```python
from build123d import *

# Parameters (mm, degrees)
SKETCH2_R           = 2.246119438
BOSS_EXTRUDE1_DEPTH = 5
SKETCH1_W           = 67
SKETCH1_H           = 30
SKETCH1_R           = 6.25
SKETCH1_R_2         = 1
BOSS_EXTRUDE3_DEPTH = 5
SKETCH8_W           = 30
SKETCH8_H           = 40
BOSS_EXTRUDE4_DEPTH = 5
SKETCH9_W           = 30
SKETCH9_H           = 40
BOSS_EXTRUDE5_DEPTH = 5
SKETCH11_W          = 30
SKETCH11_H          = 5
BOSS_EXTRUDE6_DEPTH = 40
SKETCH12_W          = 30
SKETCH12_H          = 5
BOSS_EXTRUDE7_DEPTH = 40
SKETCH13_R          = 2.195864451
CUT_EXTRUDE1_DEPTH  = 5
SKETCH14_R          = 1
CUT_EXTRUDE2_DEPTH  = 5
SKETCH15_R          = 2.070506859
CUT_EXTRUDE3_DEPTH  = 5
SKETCH16_R          = 1.962714384
CUT_EXTRUDE4_DEPTH  = 5


with BuildPart() as part:
    # Sketch2 → Boss-Extrude1 (new body)
    with BuildSketch(Plane(origin=(0, 0, 0), x_dir=(0, 0, -1), z_dir=(1, 0, 0))):
        with BuildLine():
            Line((30, 0), (0, 0))
            Line((0, 0), (0, 40))
            Line((0, 40), (7.960594487, 40))
            ThreePointArc((7.960594487, 40), (14.468438583, 30), (20.976282678, 40))
            Line((20.976282678, 40), (30, 40))
            Line((30, 40), (30, 0))
        make_face()
        with Locations((14.468438583, 24.238644745)):
            Circle(SKETCH2_R, mode=Mode.SUBTRACT)
        with Locations((6.578911504, 27.652835849)):
            Circle(SKETCH2_R, mode=Mode.SUBTRACT)
        with Locations((3.414371088, 35.645771628)):
            Circle(SKETCH2_R, mode=Mode.SUBTRACT)
        with Locations((25.875565465, 35.29271224)):
            Circle(SKETCH2_R, mode=Mode.SUBTRACT)
        with Locations((22.461374361, 27.403185161)):
            Circle(SKETCH2_R, mode=Mode.SUBTRACT)
    boss_extrude1 = extrude(amount=-BOSS_EXTRUDE1_DEPTH)

    # Sketch1 → Boss-Extrude3 (add)
    with BuildSketch(Plane(origin=(0, 0, 0), x_dir=(1, 0, 0), z_dir=(0, 1, 0))):
        with Locations((33.5, 15)):
            Rectangle(SKETCH1_W, SKETCH1_H)
        with Locations(Location((33.5, 15, 0), (0, 0, 270))):
            Circle(SKETCH1_R, mode=Mode.SUBTRACT)
        with Locations(Location((42, 23.5, 0), (0, 0, 270))):
            Circle(SKETCH1_R_2, mode=Mode.SUBTRACT)
        with Locations(Location((42, 6.5, 0), (0, 0, 270))):
            Circle(SKETCH1_R_2, mode=Mode.SUBTRACT)
        with Locations(Location((25, 6.5, 0), (0, 0, 270))):
            Circle(SKETCH1_R_2, mode=Mode.SUBTRACT)
        with Locations(Location((25, 23.5, 0), (0, 0, 270))):
            Circle(SKETCH1_R_2, mode=Mode.SUBTRACT)
        with Locations(Location((53.5, 5, 0), (0, 0, 270))):
            Circle(SKETCH1_R_2, mode=Mode.SUBTRACT)
        with Locations(Location((53.5, 25, 0), (0, 0, 270))):
            Circle(SKETCH1_R_2, mode=Mode.SUBTRACT)
        with Locations(Location((13.5, 25, 0), (0, 0, 270))):
            Circle(SKETCH1_R_2, mode=Mode.SUBTRACT)
        with Locations(Location((13.5, 5, 0), (0, 0, 270))):
            Circle(SKETCH1_R_2, mode=Mode.SUBTRACT)
    extrude(amount=BOSS_EXTRUDE3_DEPTH)

    # Mirror1: Boss-Extrude1 across plane
    add(boss_extrude1.mirror(Plane(origin=(33.5, 0, 0), x_dir=(0, 0, 1), z_dir=(1, 0, 0))))

    # Sketch8 → Boss-Extrude4 (add)
    with BuildSketch(Plane.ZY.offset(5)):
        with Locations((-15, 20)):
            Rectangle(SKETCH8_W, SKETCH8_H)
    extrude(amount=-BOSS_EXTRUDE4_DEPTH)

    # Sketch9 → Boss-Extrude5 (add)
    with BuildSketch(Plane(origin=(72, 0, 0), x_dir=(0, 0, -1), z_dir=(1, 0, 0))):
        with Locations((15, 20)):
            Rectangle(SKETCH9_W, SKETCH9_H)
    extrude(amount=-BOSS_EXTRUDE5_DEPTH)

    # Sketch11 → Boss-Extrude6 (add)
    with BuildSketch(Plane(origin=(72, 0, 0), x_dir=(0, 0, -1), z_dir=(1, 0, 0))):
        with Locations((15, 37.5)):
            Rectangle(SKETCH11_W, SKETCH11_H)
    extrude(amount=BOSS_EXTRUDE6_DEPTH)

    # Sketch12 → Boss-Extrude7 (add)
    with BuildSketch(Plane.ZY.offset(5)):
        with Locations((-15, 37.5)):
            Rectangle(SKETCH12_W, SKETCH12_H)
    extrude(amount=BOSS_EXTRUDE7_DEPTH)

    # Sketch13 → Cut-Extrude1 (cut)
    with BuildSketch(Plane(origin=(72, 0, 0), x_dir=(0, 0, -1), z_dir=(1, 0, 0))):
        with Locations((4.552108339, 18.246803651)):
            Circle(SKETCH13_R)
        with Locations((7.738751357, 11.072716755)):
            Circle(SKETCH13_R)
        with Locations((15.064893737, 8.253168149)):
            Circle(SKETCH13_R)
        with Locations((22.238980633, 11.439811167)):
            Circle(SKETCH13_R)
        with Locations((25.058529239, 18.765953547)):
            Circle(SKETCH13_R)
        with Locations((21.871886221, 25.940040443)):
            Circle(SKETCH13_R)
        with Locations((14.545743841, 28.759589048)):
            Circle(SKETCH13_R)
        with Locations((7.371656945, 25.572946031)):
            Circle(SKETCH13_R)
    extrude(amount=-CUT_EXTRUDE1_DEPTH, mode=Mode.SUBTRACT)

    # Sketch14 → Cut-Extrude2 (cut)
    with BuildSketch(Plane.XZ.offset(-35)):
        with Locations(Location((82.265636432, -14.777839144, 0), (0, 0, 270))):
            Circle(SKETCH14_R)
        with Locations(Location((85.666207992, -23.170222577, 0), (0, 0, 270))):
            Circle(SKETCH14_R)
        with Locations(Location((94.347859261, -25.744114158, 0), (0, 0, 270))):
            Circle(SKETCH14_R)
        with Locations(Location((101.77312976, -20.561321027, 0), (0, 0, 270))):
            Circle(SKETCH14_R)
        with Locations(Location((102.350639356, -11.524592123, 0), (0, 0, 270))):
            Circle(SKETCH14_R)
        with Locations(Location((95.645511544, -5.438768625, 0), (0, 0, 270))):
            Circle(SKETCH14_R)
        with Locations(Location((86.706844325, -6.886599756, 0), (0, 0, 270))):
            Circle(SKETCH14_R)
    extrude(amount=-CUT_EXTRUDE2_DEPTH, mode=Mode.SUBTRACT)

    # Sketch15 → Cut-Extrude3 (cut)
    with BuildSketch(Plane.ZY.offset(5)):
        with Locations((-15.389362422, 28.629801574)):
            Circle(SKETCH15_R)
        with Locations((-23.658210405, 24.452096347)):
            Circle(SKETCH15_R)
        with Locations((-26.55108519, 15.65105417)):
            Circle(SKETCH15_R)
        with Locations((-22.373379963, 7.382206187)):
            Circle(SKETCH15_R)
        with Locations((-13.572337785, 4.489331401)):
            Circle(SKETCH15_R)
        with Locations((-5.303489803, 8.667036629)):
            Circle(SKETCH15_R)
        with Locations((-2.410615017, 17.468078806)):
            Circle(SKETCH15_R)
        with Locations((-6.588320245, 25.736926789)):
            Circle(SKETCH15_R)
    extrude(amount=-CUT_EXTRUDE3_DEPTH, mode=Mode.SUBTRACT)

    # Sketch16 → Cut-Extrude4 (cut)
    with BuildSketch(Plane.XZ.offset(-35)):
        with Locations(Location((-39.786222938, -13.841664359, 0), (0, 0, 270))):
            Circle(SKETCH16_R)
        with Locations(Location((-36.298214509, -6.315787831, 0), (0, 0, 270))):
            Circle(SKETCH16_R)
        with Locations(Location((-28.510221767, -3.460583916, 0), (0, 0, 270))):
            Circle(SKETCH16_R)
        with Locations(Location((-20.984345239, -6.948592346, 0), (0, 0, 270))):
            Circle(SKETCH16_R)
        with Locations(Location((-18.129141325, -14.736585087, 0), (0, 0, 270))):
            Circle(SKETCH16_R)
        with Locations(Location((-21.617149754, -22.262461615, 0), (0, 0, 270))):
            Circle(SKETCH16_R)
        with Locations(Location((-29.405142495, -25.11766553, 0), (0, 0, 270))):
            Circle(SKETCH16_R)
        with Locations(Location((-36.931019024, -21.6296571, 0), (0, 0, 270))):
            Circle(SKETCH16_R)
    extrude(amount=-CUT_EXTRUDE4_DEPTH, mode=Mode.SUBTRACT)


solid = part.part
```
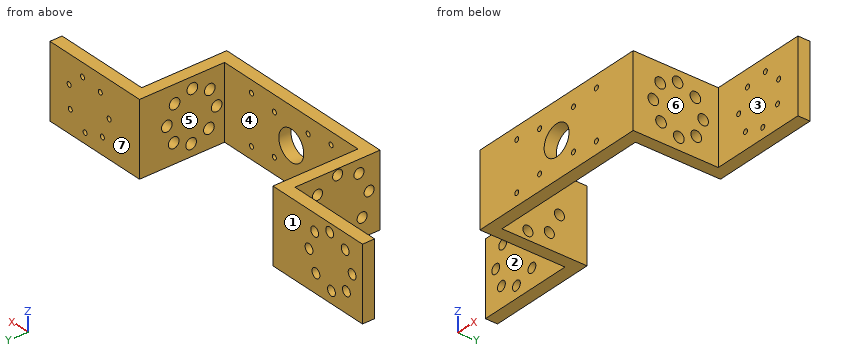
Can you work these out from the model? Positions are in its coordinate system, mm. Face numbers are marked on the shaded views. A direction names the side the tool comes from. Give positions to 0.01 mm unless a question says otherwise; leave off trailing zeros. Order: outer loops, then holes, each group sorted by start corner. A loop starts at its lowest first (then second) coordinate and runs counter-clockwise, first axis right, second up. Notation, with made-up numbers: (-36, -14) - (-11, -14) arc R30 ccw to (-11, 16) - close; hole circle Ø8 at (27, 82). An arc over 180 degrees is marked (long way). Use a Markdown table: item, result. Add a question column.
Q1. If we section it at B-B on x = 9: Write out the boundary of the cut face in (y, z), plus the area to 3 significant figures.
Q2. Please list where these lines run through material, in increasing order: line 1 along X through (y, z) = (20.5, -5.5); line 2 along Y through (x, z) = (-3.5, -3.5); line 3 along Y through (x, z) = (2.5, -8.75).
Q3. I'm going to push flat-ended pins straight in: pin 1 (4 mm diameter, centred on y = 18.25, z = -4.55, fed in from -X); pin 2 (8 mm diameter, centred on y = 4.5, z = -12.5, fed in from +X); pin 3 (2.5 mm diameter, centred on x = 101.77, z = -20.56, fed in from -Y). Where does each tip first touch, or does it pass through?
Q4. On a 3-axis mill with a long thin cutter (end or side, diameter ignored), from which of +Z, -Z, +X, -X, +Y, -Y can I reach the whole of each face in a straight line? I mean the marked faces 1, 2, 3 and 4. Say none if no direction works.
Q5. If we section it at A-A on x = 33.5: Write out the boundary of the cut face in (y, z).
Q6. If we mould it in two halves opening along X, with no side actions, what happens to the marked faces 5, 6 and 7? For each: released by +X, released by -X, zero draft, split by the parting line, or undercut.
Answers follow:
| question | item | result |
|---|---|---|
| 1 | outline | (0, -30) - (5, -30) - (5, 0) - (0, 0) - close |
| 1 | area | 150 mm^2 |
| 2 | line 1 | x = -5 to 0, 67 to 72 |
| 2 | line 2 | y = 0 to 7.65, 9.68 to 15.71, 19.23 to 40 |
| 2 | line 3 | y = 0 to 5 |
| 3 | pin 1 | stops at x = -5 |
| 3 | pin 2 | stops at x = 72 |
| 3 | pin 3 | stops at y = 35 |
| 4 | face 1 | +Z, -Z, +X, -X, +Y |
| 4 | face 2 | +Z, -Z, -X, -Y |
| 4 | face 3 | +Z, -Z, +X, -Y |
| 4 | face 4 | +Z, -Z, +Y |
| 5 | outline | (0, -30) - (5, -30) - (5, -21.25) - (0, -21.25) - close; (0, -8.75) - (5, -8.75) - (5, 0) - (0, 0) - close |
| 6 | face 5 | undercut |
| 6 | face 6 | released by +X |
| 6 | face 7 | zero draft |
